For this review, use the dimensioned drawing (mm, ordinates from the lowest corner) and the shaded views. A direction names the side the tool comes from. Round coordinates to 2 decimals unless told otherwise and drop trailing zeros. Order: outer loops, then holes, each group sorted by start corner. A loop starts at its lowest first (then second) coordinate and runs counter-clockwise, first axis right, second up. Notation, with made-up numbers: M 7,41 L 13,41 A25 ccw 13,63 Z; hole C -11.5,74 d2. An arc over 180 degrees is marked long. Use a Markdown table: item, result. Add a question column.
1. Consider section C-C on x = 57. State the section outline as (y, z) points (1 decimal).
2. For the marked faces 5 and 6, list the 3-axis set-ups (+Z, -Z, +X, -X, +Y, -Y) from which the entire face can be reached by the end or side of a thin tool; tool diameter is ignored.
3. Consider section B-B on x = 25. State the section outline as (y, z) points (1 decimal), then the cut area to 3 significant figures.
4. The part is to be moulded in two halves that separate along X. For the marked faces 1, 2, 3 and 4, say which applies: +X half, -X half, draft (parallel to the pull), parting line (faces both ways), or undercut.
5. To check wall thickness, follow probe 1 along Y at (x, z) = (10, 11.5); probe 2 along Z at (x, y) = (32, 34) (1 decimal); probe 3 along Z at (x, y) = (27, 23.5) (1 decimal). State the ranges of each line that lie inside material, in increasing order.
6. Consider section A-A on z = 42.5. State the section outline as (x, y) points.
7. Insertion check: P1, Ø8, axis at y = 41, z = 53.5, coming from the +X side (1 decimal); P2, Ø1.5, axis at x = 45, z = 33.5, coming from the -Y side; P3, Ø12, axis at y = 38, z = 12.5, coming from the -X side; P4, Ø5, axis at x = 19, y = 37.5, coming from the -Z side (1 decimal). Each pin has a flat end and moves straight along its axis. Give the tip position at first contact, or say it passes through.
8. Consider section D-D on y = 39. State the section outline as (x, z) points.
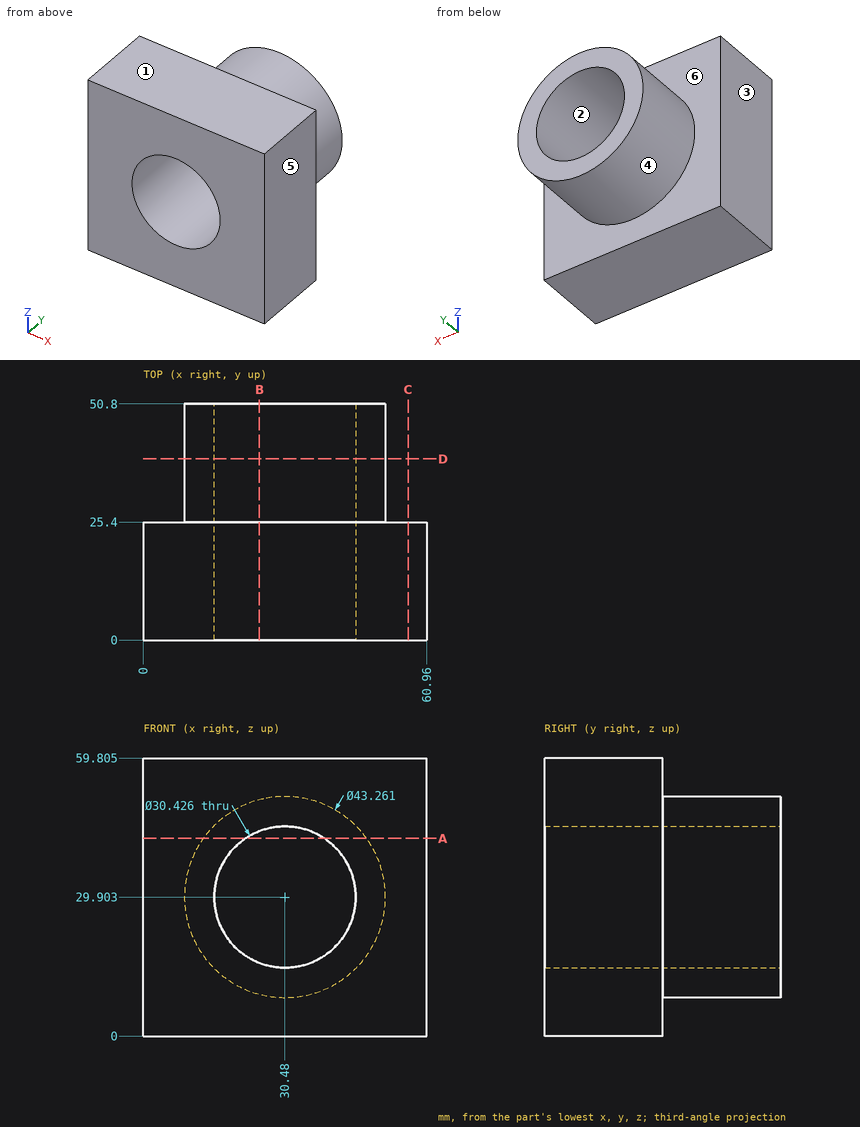
Answer block:
| question | item | result |
|---|---|---|
| 1 | outline | M 0,0 L 25.4,0 L 25.4,59.8 L 0,59.8 Z |
| 2 | face 5 | +Z, -Z, +X, +Y, -Y |
| 2 | face 6 | +Y |
| 3 | outline | M 0,0 L 25.4,0 L 25.4,9 L 50.8,9 L 50.8,15.7 L 0,15.7 Z; M 0,44.1 L 50.8,44.1 L 50.8,50.8 L 25.4,50.8 L 25.4,59.8 L 0,59.8 Z |
| 3 | area | 1,140 mm^2 |
| 4 | face 1 | draft |
| 4 | face 2 | undercut |
| 4 | face 3 | -X half |
| 4 | face 4 | parting line |
| 5 | probe 1 | 0 to 25.4 |
| 5 | probe 2 | 8.3 to 14.8, 45 to 51.5 |
| 5 | probe 3 | 0 to 15.1, 44.7 to 59.8 |
| 6 | outline | M 0,0 L 21.95,0 L 21.95,50.8 L 12.9,50.8 L 12.9,25.4 L 0,25.4 Z; M 39.01,0 L 60.96,0 L 60.96,25.4 L 48.06,25.4 L 48.06,50.8 L 39.01,50.8 Z |
| 7 | P1 | x = 39.6 |
| 7 | P2 | y = 0 |
| 7 | P3 | x = 12.1 |
| 7 | P4 | z = 10.2 |
| 8 | outline | C 30.48,29.9 d43.26; hole C 30.48,29.9 d30.43 |
